Could you check a few things on this model? Use its own coordinates, in mm. A direction names the side the tool comes from. Give positions to 0.01 mm unless a question says otherwise; leave off trailing zeros. Loops run counter-clockwise (first coordinate to the right, second up) from the corner with the lowest first, then second, coordinate; pieces in that order, holes last.
1. Imagine slicing it at A-A (x = 0). List the corners of the cut face in (y, z) for me.
2. Imagine slicing it at B-B (z = 0). List the corners of the cut face in (x, y) for me.
3. Imagine slicing it at D-D (y = 9.5). List the corners of the cut face in (x, z) for me.
4. Imagine slicing it at C-C (x = 28). List the corners of the cut face in (y, z) for me, plus the area to 3 significant figures.
5. Thinking about a two-plate mould opening in X: for faces 4 (the cylindrical face through (1.08, 0.07, -4.88)), 5 (the cylindrical face through (-20.765, 0.231, -39.923)), 6 (the flat face through (26.9, -16.5, -33.1)), 7 (the flat face through (1, 5, -9)), which applies, +X half, -X half, draft (parallel to the pull), parting line (faces both ways), or undercut?
6. For faces 1 (the flat face through (1, -5, -9)), 2 (the cylindrical face through (33.727, 10.67, 25.861)), 3 (the flat face through (26.9, 16.5, -33.1)), which set-ups out of +Z, -Z, +X, -X, +Y, -Y let a thin tool reach every point of the face, with its end or its side?
7. I need wall thicknesses on line 1 along X through (y, z) = (-14.5, -0.5); line 2 along Z through (x, y) = (0, -1.5). Which ranges of each line are inside material? Lowest first, please.
8. For P1, Ø2, axis at x = 6, y = 5.5, coming from the -Z side; P2, Ø6, axis at x = -35.5, y = 9, coming from the +Z side; P3, Ø4, axis at x = 23.5, z = -30.5, coming from the +Y side, each with a flat end and sliding along its axis, tell me the tip position at first contact or that it passes through.
Autodesk Inventor part; units mm, degrees
ref_plane "YZ Plane" through (0, 0, 0) normal (1, 0, 0) x (0, 1, 0)
ref_plane "XZ Plane" through (0, 0, 0) normal (0, 1, 0) x (-1, 0, 0)
ref_plane "XY Plane" through (0, 0, 0) normal (0, 0, 1) x (1, 0, 0)
sketch "Sketch1" plane through (0, 0, 0) normal (0, 1, 0) x (-1, 0, 0)
  circle A0 centre (0, 0) radius 42.5
  circle A1 centre (0, 0) radius 45
  circle A2 centre (0, 0) radius 5
  dimension "d0" = 85
  dimension "d3" = 90
  dimension "d6" = 10
extrude "Extrusion1" add sketch "Sketch1" along normal mid plane 10 contours A0 | A2
extrude "Extrusion2" add sketch "Sketch1" along normal mid plane 33 contours A1
extrude "Extrusion3" cut sketch "Sketch1" along normal mid plane 33 contours A2
properties part number "WheelCore"
Derived:
1. outline: (-16.5, -45) - (16.5, -45) - (16.5, -42.5) - (5, -42.5) - (5, -5) - (-5, -5) - (-5, -42.5) - (-16.5, -42.5) - close; (-16.5, 42.5) - (-5, 42.5) - (-5, 5) - (5, 5) - (5, 42.5) - (16.5, 42.5) - (16.5, 45) - (-16.5, 45) - close
2. outline: (-45, -16.5) - (-42.5, -16.5) - (-42.5, -5) - (-5, -5) - (-5, 5) - (-42.5, 5) - (-42.5, 16.5) - (-45, 16.5) - close; (5, -5) - (42.5, -5) - (42.5, -16.5) - (45, -16.5) - (45, 16.5) - (42.5, 16.5) - (42.5, 5) - (5, 5) - close
3. outline: circle Ø90 at (0, 0); hole circle Ø85 at (0, 0)
4. outline: (-16.5, -35.23) - (16.5, -35.23) - (16.5, -31.97) - (5, -31.97) - (5, 31.97) - (16.5, 31.97) - (16.5, 35.23) - (-16.5, 35.23) - (-16.5, 31.97) - (-5, 31.97) - (-5, -31.97) - (-16.5, -31.97) - close
4. area: 854 mm2
5. face 4: undercut
5. face 5: parting line
5. face 6: draft
5. face 7: undercut
6. face 1: -Y
6. face 2: +Y
6. face 3: +Z, -Z, +X, -X, +Y
7. line 1: x = -45 to -42.5, 42.5 to 45
7. line 2: z = -45 to -5, 5 to 45
8. P1: stops at z = -44.72
8. P2: stops at z = 31.12
8. P3: stops at y = 5
